```python
from build123d import *

# Parameters (mm, degrees)
SALIENTE_EXTRUIR1_START    = -22.283463782
SALIENTE_EXTRUIR1_DEPTH    = 135
SALIENTE_EXTRUIR2_START    = -15.533463782
SALIENTE_EXTRUIR2_DEPTH    = 121.5
SALIENTE_EXTRUIR2_2_DEPTH  = 3
SALIENTE_EXTRUIR2_START_2  = 102.966536218
SALIENTE_EXTRUIR2_3_DEPTH  = 3
CORTAR_EXTRUIR1_DEPTH      = 10
CORTAR_EXTRUIR1_DEPTH_BACK = 148
CHAFL_N1_SIZE              = 5
CHAFL_N1_SIZE2             = 3.934668741
CROQUIS5_W                 = 11.5
CROQUIS5_H                 = 16.108624933
SALIENTE_EXTRUIR3_DEPTH    = 8
CORTAR_EXTRUIR2_DEPTH      = 14.8
REDONDEO1_R                = 3
CROQUIS7_R                 = 2
CROQUIS7_R_2               = 3
CROQUIS7_R_3               = 1.25
SALIENTE_EXTRUIR4_DEPTH    = 5


# Read off the part's stored shape, not the designer's step: Saliente-Extruir1, Saliente-Extruir2
with BuildPart() as part:
    # Saliente-Extruir1 outline → Saliente-Extruir1 (new body)
    with BuildSketch(Plane.YZ.offset(SALIENTE_EXTRUIR1_START)):
        Polygon((-75.458190571, 5.674155302), (-73.507815836, 0), (-2.064199728, 0), (-4.014574463, 5.674155302), align=None)
    extrude(amount=SALIENTE_EXTRUIR1_DEPTH)

    # Saliente-Extruir2 outline → Saliente-Extruir2 (add)
    with BuildSketch(Plane.YZ.offset(SALIENTE_EXTRUIR2_START)):
        Polygon((-63.757815836, 0), (-66.757815836, 0), (-64.807441101, -5.674155302), (-61.807441101, -5.674155302), align=None)
    extrude(amount=SALIENTE_EXTRUIR2_DEPTH)

    # Saliente-Extruir2 2 outline → Saliente-Extruir2 2 (add)
    with BuildSketch(Plane.YZ.offset(SALIENTE_EXTRUIR2_START)):
        Polygon((-2.064199728, 0), (-63.757815836, 0), (-61.807441101, -5.674155302), (-0.113824993, -5.674155302), align=None)
    extrude(amount=SALIENTE_EXTRUIR2_2_DEPTH)

    # Saliente-Extruir2 3 outline → Saliente-Extruir2 3 (add)
    with BuildSketch(Plane.YZ.offset(SALIENTE_EXTRUIR2_START_2)):
        Polygon((-2.064199728, 0), (-63.757815836, 0), (-61.807441101, -5.674155302), (-0.113824993, -5.674155302), align=None)
    extrude(amount=SALIENTE_EXTRUIR2_3_DEPTH)

    # Croquis3 → Cortar-Extruir1 (cut, two sides: drawn at the far end of the back side and taken through both)
    with BuildSketch(Plane(origin=(105.966536218, 0, 0), x_dir=(0, 0, -1), z_dir=(1, 0, 0)).offset(-CORTAR_EXTRUIR1_DEPTH_BACK)):
        Polygon((137.63492959, 43.681305963), (7.625291737, -57.488760722), (7.625291737, -67.23888859), (-5.407688567, -80.271868893), (-9.341803419, -77.990953795), (-7.87522913, -69.550856699), (-8.264975448, -68.650724899), (138.464177577, 45.530026939), align=None)
    extrude(amount=CORTAR_EXTRUIR1_DEPTH + CORTAR_EXTRUIR1_DEPTH_BACK, mode=Mode.SUBTRACT)

    # Chaflán1
    chafl_n1_edges = [part.edges().sort_by_distance(p)[0] for p in [
        (45.216536218, -2.064199728, 0),
    ]]
    chafl_n1_side = [part.faces().sort_by_distance(p)[0] for p in [
        (45.216536218, -32.141669504, 0),
    ]]
    chamfer(chafl_n1_edges, length=CHAFL_N1_SIZE, length2=CHAFL_N1_SIZE2, reference=chafl_n1_side[0])

    # Croquis5 → Saliente-Extruir3 (add)
    with BuildSketch(Plane(origin=(0, 0, 0), x_dir=(-1, 0, 0), z_dir=(0, 0, -1))):
        with Locations((-44.930876317, -31.711417234)):
            Rectangle(CROQUIS5_W, CROQUIS5_H)
    extrude(amount=SALIENTE_EXTRUIR3_DEPTH)

    # Croquis6 → Cortar-Extruir2 (cut)
    with BuildSketch(Plane(origin=(50.680876317, 0, 0), x_dir=(0, 0, -1), z_dir=(1, 0, 0))):
        with BuildLine():
            Line((5.9, -36.7657297), (5.9, -26.657104767))
            ThreePointArc((5.9, -26.657104767), (4, -24.757104767), (2.1, -26.657104767))
            Line((2.1, -26.657104767), (2.1, -36.7657297))
            ThreePointArc((2.1, -36.7657297), (4, -38.6657297), (5.9, -36.7657297))
        make_face()
    extrude(amount=-CORTAR_EXTRUIR2_DEPTH, mode=Mode.SUBTRACT)

    # Redondeo1
    redondeo1_edges = [part.edges().sort_by_distance(p)[0] for p in [
        (44.930876317, -23.657104767, -8),
        (44.930876317, -39.7657297, -8),
    ]]
    fillet(redondeo1_edges, radius=REDONDEO1_R)

    # Croquis7 → Saliente-Extruir4 (add)
    # profile 1 of 3: a face of its own
    with BuildSketch(Plane(origin=(0, 0, 0), x_dir=(-1, 0, 0), z_dir=(0, 0, -1))):
        with Locations(Location((-84.06385674, -47.697252062, 0), (0, 0, 180))):
            Circle(CROQUIS7_R)
    # profile 2 of 3: a face of its own
    with BuildSketch(Plane(origin=(0, 0, 0), x_dir=(-1, 0, 0), z_dir=(0, 0, -1))):
        with Locations(Location((-93.07385674, -15.807252062, 0), (0, 0, 180))):
            Circle(CROQUIS7_R_2)
        with Locations((-93.07385674, -15.807252062)):
            Circle(CROQUIS7_R_3, mode=Mode.SUBTRACT)
    # profile 3 of 3: a face of its own
    with BuildSketch(Plane(origin=(0, 0, 0), x_dir=(-1, 0, 0), z_dir=(0, 0, -1))):
        with Locations(Location((-75.23385674, -15.807252062, 0), (0, 0, 180))):
            Circle(CROQUIS7_R_2)
        with Locations((-75.23385674, -15.807252062)):
            Circle(CROQUIS7_R_3, mode=Mode.SUBTRACT)
    extrude(amount=SALIENTE_EXTRUIR4_DEPTH)


solid = part.part
```
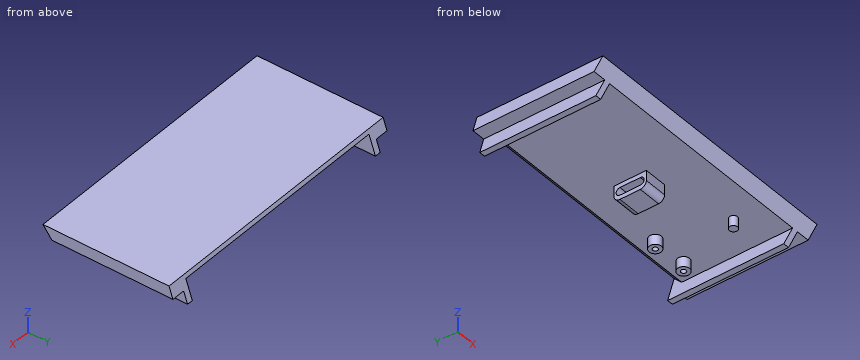
Work out the finished part from the listing and answer in its coordinate system (mm). Round coordinates to 2 decimals unless told otherwise and drop trailing zeros. Write each loop counter-clockwise with the first axis right and the second up, starting at its lowest first coordinate (ties: lowest second). Pieces come first, ordered by that corner, then holes. Notation, with made-up numbers: (-12, 32) - (32, 32) arc R23 ccw to (32, 49) - close; hole circle Ø1 at (-10.75, -14.5). An arc over 180 degrees is marked (long way). Return JSON: item names as keys, results as strings. Group by question number.
Q1. The part is cut by section A-A on z = 2.5. Write down the section's boundary in (x, y), then the cut area to 3 significant figures.
Q2. Find the intervals of material crossed by L1, parallel to X at y = -13.5, z = -1.5; L2, parallel to X at y = -31, z = -3.25; L3, parallel to Z at x = 47, y = -17.5, in increasing order.
Q3. The part is cut by section B-B on x = 15.5. Write down the section's boundary in (y, z), then the cut area to 3 significant figures.
Q4. Each of these flat-tipped pins is pushed along its axis until it touches: pin 1 Ø6.5 at (y, z) = (-29, -5) entering from -X; pin 2 Ø4 at (x, z) = (33.5, 2) entering from -Y; pin 3 Ø6 at (y, z) = (-9.5, -1.5) entering from +X; pin 4 Ø1.8 at (x, y) = (76, -15) entering from -Z. Where does it stop, or does it pass through?
Solved:
{
 "1": {"outline": "(-22.28, -64.16) - (112.72, -64.16) - (112.72, -2.92) - (102.97, -2.92) - (102.97, -4.56) - (-12.53, -4.56) - (-12.53, -2.92) - (-22.28, -2.92) - close", "area": "8,080 mm²"},
 "2": {"L1": "-15.53 to -12.53, 73.32 to 77.15, 91.16 to 94.99, 102.97 to 105.97", "L2": "-15.53 to -12.53, 102.97 to 105.97", "L3": "0 to 5.67"},
 "3": {"outline": "(-66.63, 5.67) - (-62.22, 0) - (-7.06, 0) - (-3.34, 3.72) - (-4.01, 5.67) - close", "area": "339 mm²"},
 "4": {"pin 1": "x = -15.53", "pin 2": "y = -65.33", "pin 3": "x = 112.72", "pin 4": "z = -5"}
}
